The drawing under review shows one solid part. Ordinate dimensions are in mm from its lowest x, y, z. Coordinates: 2 decimals unless noted, no trailing zeros. Loops run counter-clockwise (first coordinate to the right, second up) from the corner with the lowest first, then second, coordinate; pieces in that order, holes last.
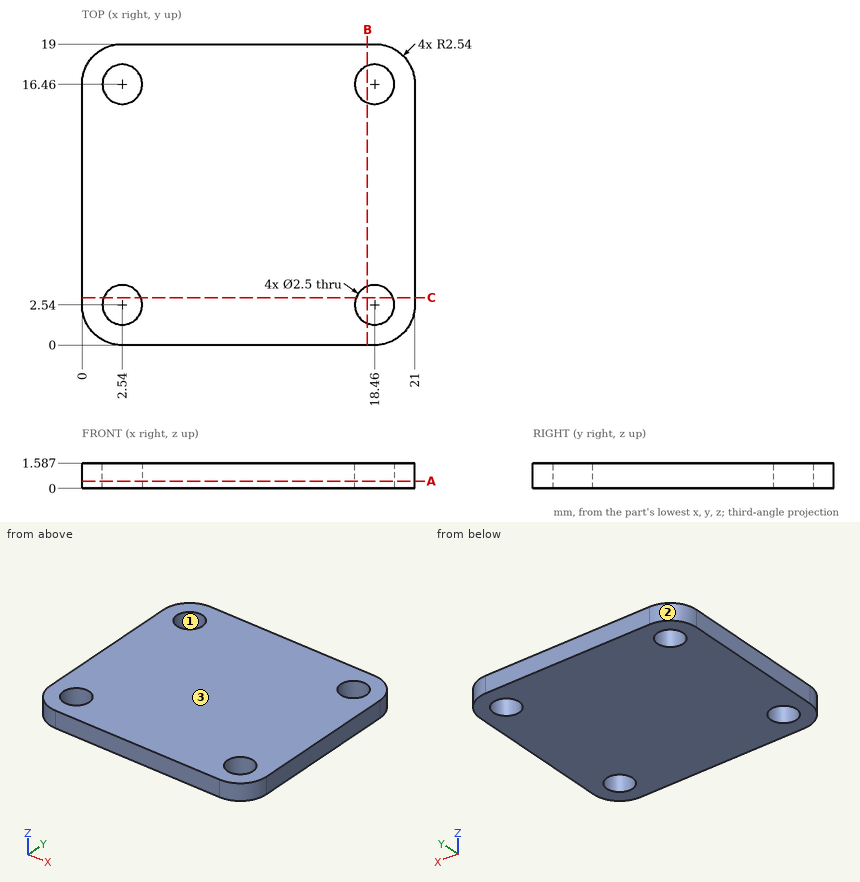
Q1. For line 1 (Y direction, x = 18.46, z = 1.05); line 2 (Y direction, x = 3.5, z = 0.5); line 3 (X direction, y = 2, z = 1.2), list the stretches that pass through material, from the lowest coordinate up.
Q2. Take a section at C-C, the plane y = 3. Write out the cut boundary in (x, z).
Q3. Take a section at B-B, the plane x = 18. Write out the cut boundary in (y, z).
Q4. The part is to be moulded in two halves that separate along X. For the marked faces 1, 2 and 3, say which applies: pulls with the +X half, pulls with the -X half, needs draft (parallel to the pull), parting line crosses it, or undercut.
Q5. Take a section at A-A, the plane z = 0.45. Write out the cut boundary in (x, y), then the cut area to 3 significant figures.
Entries:
1. line 1: y = 0 to 1.29, 3.79 to 15.21, 17.71 to 19
1. line 2: y = 0 to 1.74, 3.34 to 15.66, 17.26 to 19
1. line 3: x = 0.06 to 1.41, 3.67 to 17.33, 19.59 to 20.94
2. outline: (0, 0) - (1.38, 0) - (1.38, 1.59) - (0, 1.59) - close; (3.7, 0) - (17.3, 0) - (17.3, 1.59) - (3.7, 1.59) - close; (19.62, 0) - (21, 0) - (21, 1.59) - (19.62, 1.59) - close
3. outline: (0, 0) - (1.38, 0) - (1.38, 1.59) - (0, 1.59) - close; (3.7, 0) - (15.3, 0) - (15.3, 1.59) - (3.7, 1.59) - close; (17.62, 0) - (19, 0) - (19, 1.59) - (17.62, 1.59) - close
4. face 1: undercut
4. face 2: pulls with the -X half
4. face 3: needs draft
5. outline: (0, 2.54) arc R2.54 ccw to (2.54, 0) - (18.46, 0) arc R2.54 ccw to (21, 2.54) - (21, 16.46) arc R2.54 ccw to (18.46, 19) - (2.54, 19) arc R2.54 ccw to (0, 16.46) - close; hole circle Ø2.5 at (2.54, 2.54); hole circle Ø2.5 at (2.54, 16.46); hole circle Ø2.5 at (18.46, 2.54); hole circle Ø2.5 at (18.46, 16.46)
5. area: 374 mm2
